from build123d import *

# Parameters (mm, degrees)
CROQUIS1_W              = 90
CROQUIS1_H              = 90
SALIENTE_EXTRUIR1_DEPTH = 4
CROQUIS2_W              = 90
CROQUIS2_H              = 90
SALIENTE_EXTRUIR2_DEPTH = 25
CORTAR_EXTRUIR1_DEPTH   = 4
CORTAR_EXTRUIR1_DRAFT   = -23
CROQUIS6_W              = 10
CROQUIS6_H              = 10
SALIENTE_EXTRUIR4_DEPTH = 4
CORTAR_EXTRUIR2_START   = -8
CROQUIS7_R              = 1.625
CORTAR_EXTRUIR2_DEPTH   = 8
CORTAR_EXTRUIR3_DEPTH   = 6
CROQUIS9_R              = 1.625
CORTAR_EXTRUIR4_DEPTH   = 4
CORTAR_EXTRUIR5_DEPTH   = 2
CORTAR_EXTRUIR6_DEPTH   = 6
CROQUIS14_W             = 18.6
CROQUIS14_H             = 12.2
CORTAR_EXTRUIR7_DEPTH   = 4


with BuildPart() as part:
    # Croquis1 → Saliente-Extruir1 (new body)
    with BuildSketch(Plane.XY):
        with Locations((0.511455403, -1.711718513)):
            Rectangle(CROQUIS1_W, CROQUIS1_H)
    extrude(amount=SALIENTE_EXTRUIR1_DEPTH)

    # Croquis2 → Saliente-Extruir2 (add)
    with BuildSketch(Plane(origin=(0, 0, 0), x_dir=(-1, 0, 0), z_dir=(0, 0, -1))):
        with Locations((-0.511455403, -1.711718513)):
            Rectangle(CROQUIS2_W, CROQUIS2_H)
        Polygon((40.488544597, -27.157447779), (40.488544597, -42.711718513), (-41.511455403, -42.711718513), (-41.511455403, 39.288281487), (40.488544597, 39.288281487), align=None, mode=Mode.SUBTRACT)
    extrude(amount=SALIENTE_EXTRUIR2_DEPTH)


with BuildPart() as cortar_extruir1_tool:
    # Croquis4 → Cortar-Extruir1 (with draft: the straight prism first)
    with BuildSketch(Plane(origin=(45.511455403, 0, 0), x_dir=(0, 0, -1), z_dir=(1, 0, 0))):
        Polygon((0, -21.474747311), (0, -31.451823221), (0, -32.175243971), (7.383420942, -32.175243971), (7.383420942, -31.451823221), (7.383420942, -21.474747311), (7.383420942, -20.751326561), (0, -20.751326561), align=None)
    extrude(amount=-CORTAR_EXTRUIR1_DEPTH)
    # Cortar-Extruir1: the draft: its side faces are tilted about the plane it starts from
    cortar_extruir1_sides = [cortar_extruir1_tool.faces().sort_by_distance(p)[0] for p in [
        (43.511455403, -26.463285266, 0),
        (43.511455403, -26.463285266, -7.383420942),
        (43.511455403, -32.175243971, -3.691710471),
        (43.511455403, -20.751326561, -3.691710471),
    ]]
    draft(cortar_extruir1_sides, Plane(origin=(45.511455403, 0, 0), x_dir=(0, 0, -1), z_dir=(1, 0, 0)), CORTAR_EXTRUIR1_DRAFT)


with BuildPart() as part_1:
    add(part.part)

    # Cortar-Extruir1: cut by cortar_extruir1_tool
    add(cortar_extruir1_tool.part, mode=Mode.SUBTRACT)

    # Croquis6 → Saliente-Extruir4 (add)
    with BuildSketch(Plane(origin=(0, 0, 0), x_dir=(-1, 0, 0), z_dir=(0, 0, -1))):
        with Locations((-36.511455403, 34.288281487)):
            Rectangle(CROQUIS6_W, CROQUIS6_H)
        with Locations((-36.511455403, -37.711718513)):
            Rectangle(CROQUIS6_W, CROQUIS6_H)
        with Locations((12.157098337, -37.711718513)):
            Rectangle(CROQUIS6_W, CROQUIS6_H)
        with Locations((12.157098337, 34.288281487)):
            Rectangle(CROQUIS6_W, CROQUIS6_H)
    extrude(amount=SALIENTE_EXTRUIR4_DEPTH)

    # Croquis7 → Cortar-Extruir2 (cut)
    with BuildSketch(Plane(origin=(0, 0, -4), x_dir=(-1, 0, 0), z_dir=(0, 0, -1)).offset(CORTAR_EXTRUIR2_START)):
        with Locations((-36.511455403, 34.288281487)):
            Circle(CROQUIS7_R)
        with Locations((-36.511455403, -37.711718513)):
            Circle(CROQUIS7_R)
        with Locations((12.157098337, -37.711718513)):
            Circle(CROQUIS7_R)
        with Locations((12.157098337, 34.288281487)):
            Circle(CROQUIS7_R)
    extrude(amount=CORTAR_EXTRUIR2_DEPTH, mode=Mode.SUBTRACT)

    # Croquis8 → Cortar-Extruir3 (cut)
    with BuildSketch(Plane.XY.offset(4)):
        Polygon((36.511455403, -40.891718513), (39.265416187, -39.301718513), (39.265416187, -36.121718513), (36.511455403, -34.531718513), (33.757494619, -36.121718513), (33.757494619, -39.301718513), align=None)
        Polygon((36.511455403, 31.108281487), (39.265416187, 32.698281487), (39.265416187, 35.878281487), (36.511455403, 37.468281487), (33.757494619, 35.878281487), (33.757494619, 32.698281487), align=None)
    extrude(amount=-CORTAR_EXTRUIR3_DEPTH, mode=Mode.SUBTRACT)

    # Croquis9 → Cortar-Extruir4 (cut)
    with BuildSketch(Plane(origin=(0, 0, 0), x_dir=(-1, 0, 0), z_dir=(0, 0, -1))):
        with Locations((-35.631455403, 3.678281487)):
            Circle(CROQUIS9_R)
        with Locations((29.988544597, -1.711718513)):
            Circle(CROQUIS9_R)
    extrude(amount=-CORTAR_EXTRUIR4_DEPTH, mode=Mode.SUBTRACT)

    # Croquis10 → Cortar-Extruir5 (cut)
    with BuildSketch(Plane.XY.offset(4)):
        Polygon((-29.988544597, -4.891718513), (-27.234583813, -3.301718513), (-27.234583813, -0.121718513), (-29.988544597, 1.468281487), (-32.742505381, -0.121718513), (-32.742505381, -3.301718513), align=None)
        Polygon((35.631455403, 0.498281487), (38.385416187, 2.088281487), (38.385416187, 5.268281487), (35.631455403, 6.858281487), (32.877494619, 5.268281487), (32.877494619, 2.088281487), align=None)
    extrude(amount=-CORTAR_EXTRUIR5_DEPTH, mode=Mode.SUBTRACT)

    # Croquis11 → Cortar-Extruir6 (cut)
    with BuildSketch(Plane.XY.offset(4)):
        Polygon((-12.157098337, 31.108281487), (-9.403137553, 32.698281487), (-9.403137553, 35.878281487), (-12.157098337, 37.468281487), (-14.911059122, 35.878281487), (-14.911059122, 32.698281487), align=None)
        Polygon((-12.157098337, -34.531718513), (-14.911059122, -36.121718513), (-14.911059122, -39.301718513), (-12.157098337, -40.891718513), (-9.403137553, -39.301718513), (-9.403137553, -36.121718513), align=None)
    extrude(amount=-CORTAR_EXTRUIR6_DEPTH, mode=Mode.SUBTRACT)

    # Croquis14 → Cortar-Extruir7 (cut)
    with BuildSketch(Plane(origin=(0, 43.288281487, 0), x_dir=(1, 0, 0), z_dir=(0, 1, 0))):
        with Locations((4.864130661, 13.073723415)):
            Rectangle(CROQUIS14_W, CROQUIS14_H)
    extrude(amount=-CORTAR_EXTRUIR7_DEPTH, mode=Mode.SUBTRACT)


solid = part_1.part
Could you check a few things on this model? Use its own coordinates, in mm. A direction names the side the tool comes from. Coordinates: 2 decimals unless noted, no trailing zeros. Order: outer loops, then holes, each group sorted by start corner. A loop starts at its lowest first (then second) coordinate and runs counter-clockwise, first axis right, second up. Notation, with made-up numbers: (36.25, 43.25) - (61.25, 43.25) arc R20 cw to (61.25, 48.25) - close; hole circle Ø4 at (18.5, -31). An arc over 180 degrees is marked (long way). Answer in a Markdown table with one row per item. Add a question column.
(1) If we section it at D-D, the plane y = 16.5: Please give me the cut outline in (x, z), then the cut area to 3 significant figures.
(2) On a 3-axis mill with a long thin cutter (end or side, diameter ignored), from which of +Z, -Z, +X, -X, +Y, -Y can I reach the whole of each face in a straight line? I mean faces 1 (the face through (-28.59, 0.66, 3.01)), 2 (the face through (43.98, -21.4, -3.74)), 3 (the face through (-10, -38, -4)). Say none if no direction works.
(3) If we mould it in two halves opening along Y, with no side actions, what happens to faces 4 (the face through (-4.436, 41, -13)), 5 (the face through (31.511, -38, -2)), 6 (the face through (1, 43.288, -4)), 7 (the face through (41.511, -2, -12))? For each: released by +Y, released by -Y, zero draft, split by the parting line, or undercut.
(4) If we section it at A-A, the plane x = 7.5: Please give me the cut outline in (y, z), then the cut area to 3 significant figures.
(5) If we section it at B-B, the plane z = -23: Please give me the cut outline in (x, y), then the cut area to 3 significant figures.
(6) If we section it at C-C, the plane z = -14.25: Please give me the cut outline in (x, y), then the cut area to 3 significant figures.
(7) I need wall thicknesses on L1, parallel to X at y = -41, z = -2.5; L2, parallel to X at y = -21, z = -17.5; L3, parallel to Y at x = 24, z = -12.75. Which ranges of each line are inside material? Lowest first, please.
(8) Will these pins go through, and if not, where does the flat tip stop? pin 1 (3 mm diameter, centred on x = 36, y = 32.5, fed in from -Z); pin 2 (1.7 mm diameter, centred on x = -12, y = -39, fed in from +Z).
Results are:
| question | item | result |
|---|---|---|
| 1 | outline | (-44.49, -25) - (-40.49, -25) - (-40.49, 0) - (41.51, 0) - (41.51, -25) - (45.51, -25) - (45.51, 4) - (-44.49, 4) - close |
| 1 | area | 560 mm2 |
| 2 | face 1 | +Z |
| 2 | face 2 | +X |
| 2 | face 3 | -Z |
| 3 | face 4 | zero draft |
| 3 | face 5 | undercut |
| 3 | face 6 | released by +Y |
| 3 | face 7 | undercut |
| 4 | outline | (-46.71, -25) - (-42.71, -25) - (-42.71, 0) - (39.29, 0) - (39.29, -6.97) - (43.29, -6.97) - (43.29, 4) - (-46.71, 4) - close; (39.29, -25) - (43.29, -25) - (43.29, -19.17) - (39.29, -19.17) - close |
| 4 | area | 511 mm2 |
| 5 | outline | (-44.49, -46.71) - (45.51, -46.71) - (45.51, 43.29) - (-44.49, 43.29) - close; hole (-40.49, -42.71) - (41.51, -42.71) - (41.51, 39.29) - (-40.49, 39.29) - close |
| 5 | area | 1,380 mm2 |
| 6 | outline | (-44.49, -46.71) - (45.51, -46.71) - (45.51, 43.29) - (14.16, 43.29) - (14.16, 39.29) - (41.51, 39.29) - (41.51, -42.71) - (-40.49, -42.71) - (-40.49, 39.29) - (-4.44, 39.29) - (-4.44, 43.29) - (-44.49, 43.29) - close |
| 6 | area | 1,300 mm2 |
| 7 | L1 | x = -44.49 to -40.49, -17.16 to -7.16, 31.51 to 45.51 |
| 7 | L2 | x = -44.49 to -40.49, 41.51 to 45.51 |
| 7 | L3 | y = -46.71 to -42.71, 39.29 to 43.29 |
| 8 | pin 1 | stops at z = -4 |
| 8 | pin 2 | stops at z = -2 |
